Model file for the job. Use its own axes, mm. Round coordinates to 2 decimals unless told otherwise and drop trailing zeros. Loops run counter-clockwise (first coordinate to the right, second up) from the corner with the lowest first, then second, coordinate; pieces in that order, holes last.
Autodesk Fusion 360 part; units mm, degrees
sketch "Sketch1" plane through (0, 0, 0) normal (0, 0, 1) x (1, 0, 0)
  circle A0 centre (-75, 75) radius 1.75
  circle A1 centre (-75, -75) radius 1.75
  circle A2 centre (75, -75) radius 1.75
  circle A3 centre (75, 75) radius 1.75
  circle A4 centre (0, 0) radius 132
  circle A5 centre (0, 0) radius 12.5
  dimension "d1" = 264
  dimension "d4" = 3.5
  dimension "d6" = 360
  dimension "d46" = 75
  dimension "d47" = 75
  dimension "d48" = 25
extrude "Extrude1" add sketch "Sketch1" along normal blind 3
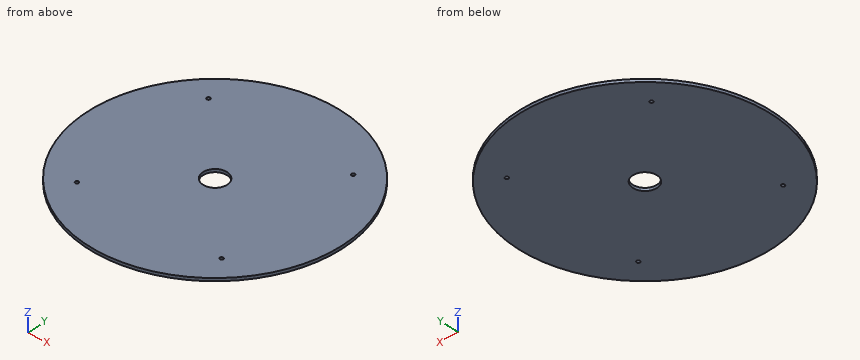
Q1. Slice it at A-A on x = 0. Give the cut face in (y, z), plus the area to 3 significant figures.
Q2. Slice it at B-B on z = 2.4. Give the cut face in (x, y), plus the area to 3 significant figures.
Q3. Slice it at D-D on x = -69. Give the cut face in (y, z), plus the area to 3 significant figures.
Q4. Probe line 1 (Y direction, x = -75, z = 2.25); line 2 (Y direction, x = 2, z = 1.1). List the from-to ranges inside material, lowest first.
Q5. Slice it at C-C on y = 112. Give the cut face in (x, z).
Reply:
1. outline: (-132, 0) - (-12.5, 0) - (-12.5, 3) - (-132, 3) - close; (12.5, 0) - (132, 0) - (132, 3) - (12.5, 3) - close
1. area: 717 mm2
2. outline: circle Ø264 at (0, 0); hole circle Ø3.5 at (-75, -75); hole circle Ø3.5 at (-75, 75); hole circle Ø25 at (0, 0); hole circle Ø3.5 at (75, -75); hole circle Ø3.5 at (75, 75)
2. area: 54,200 mm2
3. outline: (-112.53, 0) - (112.53, 0) - (112.53, 3) - (-112.53, 3) - close
3. area: 675 mm2
4. line 1: y = -108.62 to -76.75, -73.25 to 73.25, 76.75 to 108.62
4. line 2: y = -131.98 to -12.34, 12.34 to 131.98
5. outline: (-69.86, 0) - (69.86, 0) - (69.86, 3) - (-69.86, 3) - close
